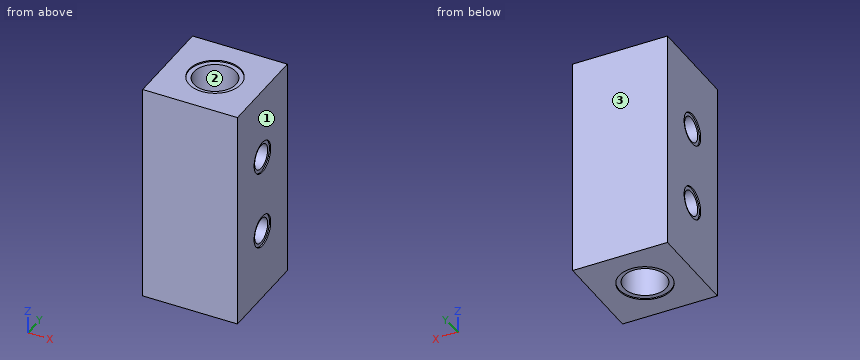
```python
from build123d import *

# Parameters (mm, degrees)
SKETCH1_W           = 38.1
SKETCH1_H           = 38.1
SKETCH1_R           = 8.509
BOSS_EXTRUDE1_DEPTH = 44.45
SKETCH2_R           = 4.953
CUT_EXTRUDE1_DEPTH  = 39.1
CUT_EXTRUDE2_START  = 44.45
SKETCH13_R          = 10.414
CUT_EXTRUDE2_DEPTH  = 0.508
CUT_EXTRUDE3_START  = -44.45
SKETCH13_2_R        = 10.414
CUT_EXTRUDE3_DEPTH  = 0.508
CUT_EXTRUDE4_START  = 19.05
SKETCH14_R          = 6.35
CUT_EXTRUDE4_DEPTH  = 0.508
CUT_EXTRUDE5_START  = 19.05
SKETCH14_3_R        = 6.35
CUT_EXTRUDE5_DEPTH  = 0.508
CUT_EXTRUDE6_START  = -19.05
SKETCH14_4_R        = 6.35
CUT_EXTRUDE6_DEPTH  = 0.508


with BuildPart() as part:
    # Sketch1 → Boss-Extrude1 (new body, symmetric)
    with BuildSketch(Plane.XY):
        Rectangle(SKETCH1_W, SKETCH1_H)
        Circle(SKETCH1_R, mode=Mode.SUBTRACT)
    extrude(amount=BOSS_EXTRUDE1_DEPTH, both=True)

    # Sketch2 → Cut-Extrude1 (cut, through all)
    with BuildSketch(Plane(origin=(19.05, 0, 0), x_dir=(0, 0, -1), z_dir=(1, 0, 0))):
        with Locations((-15.875, 0)):
            Circle(SKETCH2_R)
        with Locations((15.875, 0)):
            Circle(SKETCH2_R)
    extrude(amount=-CUT_EXTRUDE1_DEPTH, mode=Mode.SUBTRACT)

    # Sketch13 → Cut-Extrude2 (cut)
    with BuildSketch(Plane.XY.offset(CUT_EXTRUDE2_START)):
        Circle(SKETCH13_R)
    extrude(amount=-CUT_EXTRUDE2_DEPTH, mode=Mode.SUBTRACT)

    # Sketch13<2> → Cut-Extrude3 (cut)
    with BuildSketch(Plane.XY.offset(CUT_EXTRUDE3_START)):
        Circle(SKETCH13_2_R)
    extrude(amount=CUT_EXTRUDE3_DEPTH, mode=Mode.SUBTRACT)

    # Sketch14 → Cut-Extrude4 (cut)
    with BuildSketch(Plane(origin=(0, 0, 0), x_dir=(0, 0, -1), z_dir=(1, 0, 0)).offset(CUT_EXTRUDE4_START)):
        with Locations((-15.875, 0)):
            Circle(SKETCH14_R)
    extrude(amount=-CUT_EXTRUDE4_DEPTH, mode=Mode.SUBTRACT)

    # Sketch14<3> → Cut-Extrude5 (cut)
    with BuildSketch(Plane(origin=(0, 0, 0), x_dir=(0, 0, -1), z_dir=(1, 0, 0)).offset(CUT_EXTRUDE5_START)):
        with Locations((-15.875, 0)):
            Circle(SKETCH14_3_R)
        with Locations((15.875, 0)):
            Circle(SKETCH14_3_R)
    extrude(amount=-CUT_EXTRUDE5_DEPTH, mode=Mode.SUBTRACT)

    # Sketch14<4> → Cut-Extrude6 (cut)
    with BuildSketch(Plane(origin=(0, 0, 0), x_dir=(0, 0, -1), z_dir=(1, 0, 0)).offset(CUT_EXTRUDE6_START)):
        with Locations((-15.875, 0)):
            Circle(SKETCH14_4_R)
        with Locations((15.875, 0)):
            Circle(SKETCH14_4_R)
    extrude(amount=CUT_EXTRUDE6_DEPTH, mode=Mode.SUBTRACT)


solid = part.part
```
Check sheet for the modelled part. Datum: model origin and axes. Units: mm. Face numbers are marked on the shaded views. Round coordinates to 2 decimals unless told otherwise and drop trailing zeros. Loops run counter-clockwise (first coordinate to the right, second up) from the corner with the lowest first, then second, coordinate; pieces in that order, holes last. Notation, with made-up numbers: (-25, 20) - (11, 20) arc R33 cw to (11, 57) - close; hole circle Ø5 at (56, -20.75). An arc over 180 degrees is marked (long way). Answer as a JSON object with one key per item and string values. Group by question number.
Q1. Sectioned sample at C-C, the plane x = 16. Enter the section's corners in (y, z) (3 decimals), plus the area to 3 significant figures.
Q2. Sectioned sample at B-B, the plane z = 23.5. Enter the section's corners in (x, y), plus the area to 3 significant figures.
Q3. Scan lines: line 1 along Z through (x, y) = (15, 0); line 2 along Z through (x, y) = (10, 0); line 3 along Y through (x, z) = (0, -44.3). Record each from-to range of solid material in increasing order. Write a range as [from, to].
Q4. Sectioned sample at D-D, the plane z = -15.5. Enter the section's corners in (x, y).
Q5. Sectioned sample at A-A, the plane x = 0. Enter the section's corners in (y, z), plus the area to 3 significant figures.
Q6. Mould release check, pull along X, two halves, no side actions. Record for the marked faces 1, 2 and 3: released by +X, released by -X, zero draft, split by the parting line, or undercut.
Q7. Gauge pin test, flat ends, axial feed: P1, Ø11.5, axis at y = 0, z = 15.875, coming from the -X side; P2, Ø2, axis at y = -3.5, z = 13, coming from the +X side. Record the tip position at first contact, or that the pin passes through.
Solution:
{
 "1": {"outline": "(-19.05, -44.45) - (19.05, -44.45) - (19.05, 44.45) - (-19.05, 44.45) - close; hole circle Ø9.906 at (0, -15.875); hole circle Ø9.906 at (0, 15.875)", "area": "3,230 mm²"},
 "2": {"outline": "(-19.05, -19.05) - (19.05, -19.05) - (19.05, 19.05) - (-19.05, 19.05) - close; hole circle Ø17.02 at (0, 0)", "area": "1,220 mm²"},
 "3": {"line 1": "z = [-44.45, -20.83], [-10.92, 10.92], [20.83, 44.45]", "line 2": "z = [-43.94, -20.83], [-10.92, 10.92], [20.83, 43.94]", "line 3": "y = [-19.05, -10.41], [10.41, 19.05]"},
 "4": {"outline": "(-19.05, -19.05) - (19.05, -19.05) - (19.05, -6.34) - (18.54, -6.34) - (18.54, -4.94) - (6.93, -4.94) arc R8.51 cw to (-6.93, -4.94) - (-18.54, -4.94) - (-18.54, -6.34) - (-19.05, -6.34) - close; (-19.05, 6.34) - (-18.54, 6.34) - (-18.54, 4.94) - (-6.93, 4.94) arc R8.51 cw to (6.93, 4.94) - (18.54, 4.94) - (18.54, 6.34) - (19.05, 6.34) - (19.05, 19.05) - (-19.05, 19.05) - close"},
 "5": {"outline": "(-19.05, -44.45) - (-10.41, -44.45) - (-10.41, -43.94) - (-8.51, -43.94) - (-8.51, 43.94) - (-10.41, 43.94) - (-10.41, 44.45) - (-19.05, 44.45) - close; (8.51, -43.94) - (10.41, -43.94) - (10.41, -44.45) - (19.05, -44.45) - (19.05, 44.45) - (10.41, 44.45) - (10.41, 43.94) - (8.51, 43.94) - close", "area": "1,870 mm²"},
 "6": {"face 1": "released by +X", "face 2": "undercut", "face 3": "zero draft"},
 "7": {"P1": "stops at x = -18.54", "P2": "stops at x = 18.54"}
}
